Can you work these out from the model? Positions are in its coordinate system, mm. Give positions to 0.01 mm unless a question says otherwise; leave off trailing zeros. Order: outer loops, then holes, each group sorted by start corner. A loop starts at its lowest first (then second) coordinate and runs counter-clockwise, first axis right, second up. Notation, with made-up numbers: M 15,15.25 L 32,15.25 A20 ccw 32,27.25 Z; hole C 38,-30 d3. An arc over 180 degrees is marked long. Use a Markdown table: item, result. Add a question column.
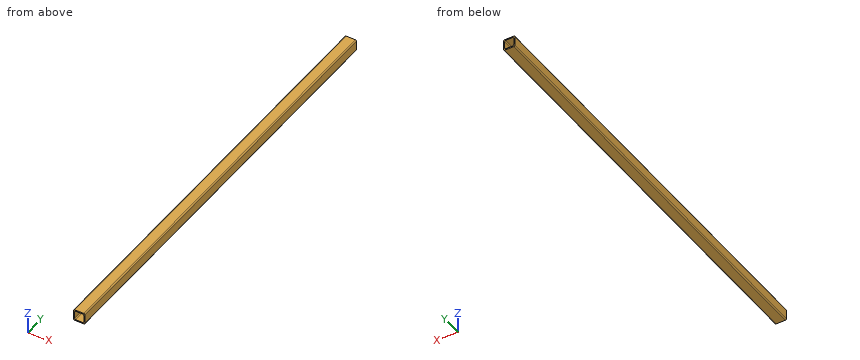
from build123d import *

# Parameters (mm, degrees)
BOSS_EXTRUDE1_START = -2175.918735
BOSS_EXTRUDE1_DEPTH = 379.319789155


with BuildPart() as part:
    # Sketch1 → Boss-Extrude1 (new body)
    with BuildSketch(Plane(origin=(0, 0, 0), x_dir=(1, 0, 0), z_dir=(0, 1, 0)).offset(BOSS_EXTRUDE1_START)):
        with BuildLine():
            Line((-51.887039023, -1.543455886), (-43.887039023, -1.543455886))
            ThreePointArc((-43.887039023, -1.543455886), (-43.179932241, -1.836349105), (-42.887039023, -2.543455886))
            Line((-42.887039023, -2.543455886), (-42.887039023, -10.543455886))
            ThreePointArc((-42.887039023, -10.543455886), (-43.179932241, -11.250562667), (-43.887039023, -11.543455886))
            Line((-43.887039023, -11.543455886), (-51.887039023, -11.543455886))
            ThreePointArc((-51.887039023, -11.543455886), (-52.594145804, -11.250562667), (-52.887039023, -10.543455886))
            Line((-52.887039023, -10.543455886), (-52.887039023, -2.543455886))
            ThreePointArc((-52.887039023, -2.543455886), (-52.594145804, -1.836349105), (-51.887039023, -1.543455886))
        make_face()
        with BuildLine():
            Line((-50.887039023, -2.543455886), (-44.887039023, -2.543455886))
            ThreePointArc((-44.887039023, -2.543455886), (-44.179932241, -2.836349105), (-43.887039023, -3.543455886))
            Line((-43.887039023, -3.543455886), (-43.887039023, -9.543455886))
            ThreePointArc((-43.887039023, -9.543455886), (-44.179932241, -10.250562667), (-44.887039023, -10.543455886))
            Line((-44.887039023, -10.543455886), (-50.887039023, -10.543455886))
            ThreePointArc((-50.887039023, -10.543455886), (-51.594145804, -10.250562667), (-51.887039023, -9.543455886))
            Line((-51.887039023, -9.543455886), (-51.887039023, -3.543455886))
            ThreePointArc((-51.887039023, -3.543455886), (-51.594145804, -2.836349105), (-50.887039023, -2.543455886))
        make_face(mode=Mode.SUBTRACT)
    extrude(amount=-BOSS_EXTRUDE1_DEPTH)


solid = part.part
1. If we section it at B-B, the plane y = -2428: List the corners of the cut face in (x, z) for me.
2. If we section it at A-A, the plane z = 6.5: List the corners of the cut face in (x, y) for me, then the cut area to 3 significant figures.
3. I need wall thicknesses on L1, parallel to X at y = -2293, z = 4.75; L2, parallel to Z at x = -44.75, y = -2453; L3, parallel to Z at x = -49.5, y = -2341. Which ranges of each line are inside material? Lowest first, please. Write a range as [from, to].
4. If we section it at C-C, the plane x = -48.5: List the corners of the cut face in (y, z) for me.
Geometry results:
| question | item | result |
|---|---|---|
| 1 | outline | M -52.89,2.54 A1 ccw -51.89,1.54 L -43.89,1.54 A1 ccw -42.89,2.54 L -42.89,10.54 A1 ccw -43.89,11.54 L -51.89,11.54 A1 ccw -52.89,10.54 Z; hole M -51.89,3.54 A1 ccw -50.89,2.54 L -44.89,2.54 A1 ccw -43.89,3.54 L -43.89,9.54 A1 ccw -44.89,10.54 L -50.89,10.54 A1 ccw -51.89,9.54 Z |
| 2 | outline | M -52.89,-2555.24 L -51.89,-2555.24 L -51.89,-2175.92 L -52.89,-2175.92 Z; M -43.89,-2555.24 L -42.89,-2555.24 L -42.89,-2175.92 L -43.89,-2175.92 Z |
| 2 | area | 759 mm^2 |
| 3 | L1 | x = [-52.89, -51.89], [-43.89, -42.89] |
| 3 | L2 | z = [1.54, 2.55], [10.53, 11.54] |
| 3 | L3 | z = [1.54, 2.54], [10.54, 11.54] |
| 4 | outline | M -2555.24,1.54 L -2175.92,1.54 L -2175.92,2.54 L -2555.24,2.54 Z; M -2555.24,10.54 L -2175.92,10.54 L -2175.92,11.54 L -2555.24,11.54 Z |
